```python
from build123d import *

# Parameters (mm, degrees)
F1_DEPTH = 3.5
F2_R     = 3.5
F3_DEPTH = 6
F4_R     = 1.5
F5_DEPTH = 29.001


with BuildPart() as f1:
    # F0 (on Top) → F1 (new body, symmetric)
    with BuildSketch(Plane.XY):
        with BuildLine():
            Line((0, -1.75), (0, 0))
            Line((0, 0), (33.5, 0))
            ThreePointArc((33.5, 0), (33.8535533906, 0.1464466094), (34, 0.5))
            Line((34, 0.5), (34, 11.35))
            ThreePointArc((34, 11.35), (34.1903805922, 11.8096194078), (34.65, 12))
            Line((34.65, 12), (34.85, 12))
            ThreePointArc((34.85, 12), (35.3096194078, 11.8096194078), (35.5, 11.35))
            Line((35.5, 11.35), (35.5, -1.75))
            Line((35.5, -1.75), (34.1035533906, -1.75))
            ThreePointArc((34.1035533906, -1.75), (33.8725835075, -1.9043291419), (33.9267766953, -2.1767766953))
            Line((33.9267766953, -2.1767766953), (36.6767766953, -4.9267766953))
            ThreePointArc((36.6767766953, -4.9267766953), (36.7578825325, -4.9809698831), (36.8535533906, -5))
            Line((36.8535533906, -5), (38.85, -5))
            ThreePointArc((38.85, -5), (39.3096194078, -4.8096194078), (39.5, -4.35))
            Line((39.5, -4.35), (39.5, -3.9))
            ThreePointArc((39.5, -3.9), (39.6903805922, -3.4403805922), (40.15, -3.25))
            Line((40.15, -3.25), (40.35, -3.25))
            ThreePointArc((40.35, -3.25), (40.8096194078, -3.0596194078), (41, -2.6))
            Line((41, -2.6), (41, 1.6))
            ThreePointArc((41, 1.6), (40.8096194078, 2.0596194078), (40.35, 2.25))
            Line((40.35, 2.25), (40.15, 2.25))
            ThreePointArc((40.15, 2.25), (39.6903805922, 2.0596194078), (39.5, 1.6))
            Line((39.5, 1.6), (39.5, -1.1))
            ThreePointArc((39.5, -1.1), (39.3096194078, -1.5596194078), (38.85, -1.75))
            Line((38.85, -1.75), (37.5, -1.75))
            Line((37.5, -1.75), (37.5, 11.96))
            ThreePointArc((37.5, 11.96), (37.5117157288, 11.9882842712), (37.54, 12))
            Line((37.54, 12), (88, 12))
            Line((88, 12), (88, 18))
            Line((88, 18), (-19, 18))
            Line((-19, 18), (-19, 12))
            Line((-19, 12), (-12, 12))
            Line((-12, 12), (-12, -4.35))
            ThreePointArc((-12, -4.35), (-11.8096194078, -4.8096194078), (-11.35, -5))
            Line((-11.35, -5), (-0.3535533906, -5))
            ThreePointArc((-0.3535533906, -5), (-0.2578825325, -4.9809698831), (-0.1767766953, -4.9267766953))
            Line((-0.1767766953, -4.9267766953), (2.5732233047, -2.1767766953))
            ThreePointArc((2.5732233047, -2.1767766953), (2.6274164925, -1.9043291419), (2.3964466094, -1.75))
            Line((2.3964466094, -1.75), (0, -1.75))
        make_face()
    extrude(amount=F1_DEPTH, both=True)

    # F2 (on face) → F3 (join)
    with BuildSketch(Plane(origin=(0, 18, 0), x_dir=(-1, 0, 0), z_dir=(0, 1, 0))):
        with Locations((-84.5, 0)):
            Circle(F2_R)
        with Locations((15.5, 0)):
            Circle(F2_R)
    extrude(amount=F3_DEPTH)

    # F4 (on face) → F5 (cut, through all)
    with BuildSketch(Plane(origin=(0, 24, 0), x_dir=(-1, 0, 0), z_dir=(0, 1, 0))):
        with Locations((-84.5, 0)):
            Circle(F4_R)
        with Locations((15.5, 0)):
            Circle(F4_R)
    extrude(amount=-F5_DEPTH, mode=Mode.SUBTRACT)


solid = f1.part
```
Verification items for the finished model (mm, model axes). A direction names the side the tool comes from. Give positions to 0.01 mm unless a question says otherwise; leave off trailing zeros. Order: outer loops, then holes, each group sorted by start corner. A loop starts at its lowest first (then second) coordinate and runs counter-clockwise, first axis right, second up. Notation, with made-up numbers: M -6.5,74 L 11.5,74 A24 ccw 11.5,93 Z; hole C 85,-11.75 d5. An arc over 180 degrees is marked long. Answer in a Markdown table with one row per item. Add a question column.
Item 1: Section check B-B, the plane y = 17. Enter the section's corners in (x, z).
Item 2: Section check D-D, the plane x = 72. Enter the section's corners in (y, z).
Item 3: Section check A-A, the plane y = 7.5. Enter the section's corners in (x, z), and give its area (3 significant figures).
Item 4: Scan lines: probe 1 along Y at (x, z) = (39, -3); probe 2 along Z at (x, y) = (-15.5, 19.5); probe 3 along X at (y, z) = (22, -0.5). Record each from-to range of solid material in increasing order. Write a range as from..to.
Item 5: Section check C-C, the plane x = 17. Enter the section's corners in (y, z).
Item 6: Mould release check, pull along Z, two halves, no side actions. Record for faces 1 (the flat face through (85, 24, -2)), 2 (the cylindrical face through (81.267, 20.958, -1.341)), 3 (the cylindrical face through (83, 18, 0)): released by +Z, released by -Z, zero draft, split by the parting line, or undercut.
Item 7: Tool access check on faces 4 (the flat face through (-18, 18, -3)), 5 (the flat face through (88, 15, 0)), 6 (the flat face through (37.5, 5, 0)), 7 (the flat face through (-12, 4, 0)), 8 (the flat face through (-18, 18, 3)). Record the directions out of +Z, -Z, +X, -X, +Y, -Y that give a thin tool (end or side, any length) a straight path to the whole face; none if there is none.
Item 8: Gauge pin test, flat ends, axial feed: pin 1 (0.7 mm diameter, centred on x = 34.5, z = -0.5, fed in from +Y); pin 2 (3.5 mm diameter, centred on y = -1, z = 1.5, fed in from +X); pin 3 (0.5 mm diameter, centred on y = -4, z = 1, fed in from +X). Record the tip position at first contact, or that the pin passes through.
Filled sheet:
| question | item | result |
|---|---|---|
| 1 | outline | M -19,-3.5 L 88,-3.5 L 88,3.5 L -19,3.5 Z; hole C -15.5,0 d3; hole C 84.5,0 d3 |
| 2 | outline | M 12,-3.5 L 18,-3.5 L 18,3.5 L 12,3.5 Z |
| 3 | outline | M -12,-3.5 L 34,-3.5 L 34,3.5 L -12,3.5 Z; M 35.5,-3.5 L 37.5,-3.5 L 37.5,3.5 L 35.5,3.5 Z |
| 3 | area | 336 mm^2 |
| 4 | probe 1 | y = -4.98..-1.73, 12..18 |
| 4 | probe 2 | z = -3.5..-1.5, 1.5..3.5 |
| 4 | probe 3 | x = -18.96..-16.91, -14.09..-12.04, 81.04..83.09, 85.91..87.96 |
| 5 | outline | M 0,-3.5 L 18,-3.5 L 18,3.5 L 0,3.5 Z |
| 6 | face 1 | zero draft |
| 6 | face 2 | split by the parting line |
| 6 | face 3 | undercut |
| 7 | face 4 | -Z, -X, +Y |
| 7 | face 5 | +Z, -Z, +X, +Y, -Y |
| 7 | face 6 | +Z, -Z |
| 7 | face 7 | +Z, -Z, -X, -Y |
| 7 | face 8 | +Z, -X, +Y |
| 8 | pin 1 | stops at y = 18 |
| 8 | pin 2 | stops at x = 41 |
| 8 | pin 3 | stops at x = 39.52 |
